```python
from build123d import *

# Parameters (mm, degrees)
SKETCH1_R           = 12.7
BOSS_EXTRUDE1_DEPTH = 3.175


with BuildPart() as part:
    # Sketch1 → Boss-Extrude1 (new body)
    with BuildSketch(Plane(origin=(0, 0, 0), x_dir=(1, 0, 0), z_dir=(0, 1, 0))):
        with BuildLine():
            Line((-18.783553311, -3.175), (-22.86, -3.175))
            Line((-22.86, -3.175), (-22.86, 3.175))
            Line((-22.86, 3.175), (-18.783553311, 3.175))
            ThreePointArc((-18.783553311, 3.175), (-13.470384182, 13.470384182), (-3.175, 18.783553311))
            Line((-3.175, 18.783553311), (-3.175, 22.86))
            Line((-3.175, 22.86), (3.175, 22.86))
            Line((3.175, 22.86), (3.175, 18.783553311))
            ThreePointArc((3.175, 18.783553311), (13.470384182, 13.470384182), (18.783553311, 3.175))
            Line((18.783553311, 3.175), (22.86, 3.175))
            Line((22.86, 3.175), (22.86, -3.175))
            Line((22.86, -3.175), (18.783553311, -3.175))
            ThreePointArc((18.783553311, -3.175), (13.470384182, -13.470384182), (3.175, -18.783553311))
            Line((3.175, -18.783553311), (3.175, -22.86))
            Line((3.175, -22.86), (-3.175, -22.86))
            Line((-3.175, -22.86), (-3.175, -18.783553311))
            ThreePointArc((-3.175, -18.783553311), (-13.470384182, -13.470384182), (-18.783553311, -3.175))
        make_face()
        Circle(SKETCH1_R, mode=Mode.SUBTRACT)
    extrude(amount=BOSS_EXTRUDE1_DEPTH)


solid = part.part
```
Here's how the part is built. I have some questions about the finished solid (model axes, mm). A direction names the side the tool comes from. Coordinates: 2 decimals unless noted, no trailing zeros. Order: outer loops, then holes, each group sorted by start corner. A loop starts at its lowest first (then second) coordinate and runs counter-clockwise, first axis right, second up. Notation, with made-up numbers: M 81.25,23 L 123.25,23 A19 cw 123.25,40 Z; hole C 80.5,-34.5 d7. An arc over 180 degrees is marked long. Answer as a JSON object with one key per item and string values. Group by question number.
(1) I need wall thicknesses on probe 1 along X at (y, z) = (1.4, 0); probe 2 along X at (y, z) = (2.1, -4). Which ranges of each line are inside material? Lowest first, please.
(2) If we mould it in two halves opening along X, with no side actions, what happens to faces 4 (the face through (-13.59, 1.57, -13.35)), 5 (the face through (-2.75, 1.57, 12.4)), 6 (the face through (-21, 2, -3.175))? For each: released by +X, released by -X, zero draft, split by the parting line, or undercut.
(3) Suppose I cut it at B-B, the plane z = 0. Please give me the cut outline in (x, y) (3 decimals), then the cut area to 3 significant figures.
(4) Which directions (+Z, -Z, +X, -X, +Y, -Y) give clear straight access to the entire face, cutting with the end or side of a thin tool? Please do faces 1 (the face through (21, 2, -3.175)), 2 (the face through (-3.175, 2, 21)), 3 (the face through (21, 2, 3.175)).
(5) For pin 1 (1.5 mm diameter, centred on y = 0.5, z = -18, fed in from +X); pin 2 (3 mm diameter, centred on x = -10.5, z = -13.5, fed in from -Y); pin 3 (1.6 mm diameter, centred on x = 21, y = 2, fed in from -Z) (3 decimals); pin 4 (23 mm diameter, centred on x = 0, z = 0, fed in from +Y), each with a flat end and sliding along its axis, tell me the tip position at first contact or that it passes through.
(6) Suppose I cut it at D-D, the plane z = -17. Please give me the cut outline in (x, y) (3 decimals), then the cut area to 3 significant figures.
(7) Suppose I cut it at C-C, the plane y = 2.4. Please give me the cut outline in (x, z) (3 decimals), then the cut area to 3 significant figures.
(8) Suppose I cut it at A-A, the plane x = 0. Please give me the cut outline in (y, z) (3 decimals).
Values found:
{
 "1": {"probe 1": "x = -22.86 to -12.7, 12.7 to 22.86", "probe 2": "x = -18.63 to -12.05, 12.05 to 18.63"},
 "2": {"face 4": "released by -X", "face 5": "undercut", "face 6": "zero draft"},
 "3": {"outline": "M -22.86,0 L -12.7,0 L -12.7,3.175 L -22.86,3.175 Z; M 12.7,0 L 22.86,0 L 22.86,3.175 L 12.7,3.175 Z", "area": "64.5 mm^2"},
 "4": {"face 1": "-Z, +X, +Y, -Y", "face 2": "+Z, -X, +Y, -Y", "face 3": "+Z, +X, +Y, -Y"},
 "5": {"pin 1": "stops at x = 8.08", "pin 2": "stops at y = 0", "pin 3": "stops at z = -3.175", "pin 4": "passes through"},
 "6": {"outline": "M -8.597,0 L 8.597,0 L 8.597,3.175 L -8.597,3.175 Z", "area": "54.6 mm^2"},
 "7": {"outline": "M -22.86,-3.175 L -18.784,-3.175 A19.05 ccw -3.175,-18.784 L -3.175,-22.86 L 3.175,-22.86 L 3.175,-18.784 A19.05 ccw 18.784,-3.175 L 22.86,-3.175 L 22.86,3.175 L 18.784,3.175 A19.05 ccw 3.175,18.784 L 3.175,22.86 L -3.175,22.86 L -3.175,18.784 A19.05 ccw -18.784,3.175 L -22.86,3.175 Z; hole C 0,0 d25.4", "area": "732 mm^2"},
 "8": {"outline": "M 0,-22.86 L 3.175,-22.86 L 3.175,-12.7 L 0,-12.7 Z; M 0,12.7 L 3.175,12.7 L 3.175,22.86 L 0,22.86 Z"}
}
